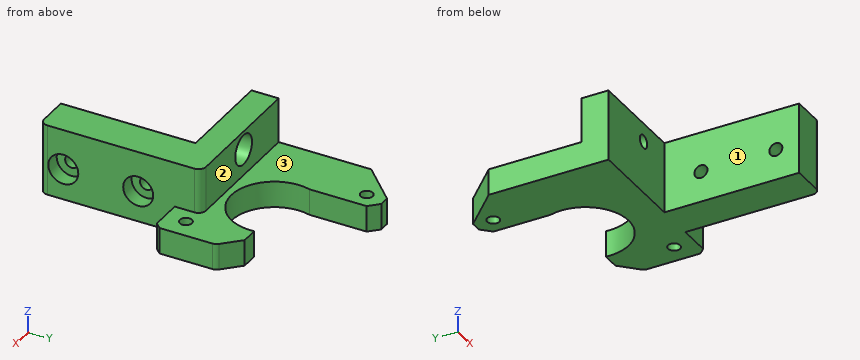
from build123d import *

# Parameters (mm, degrees)
BOSS_EXTRUDE1_DEPTH = 19
BOSS_EXTRUDE2_DEPTH = 7
SKETCH3_R           = 1.75
CUT_EXTRUDE1_DEPTH  = 37.75
SKETCH6_R           = 4
CUT_EXTRUDE4_DEPTH  = 4
SKETCH7_R           = 1.625
CUT_EXTRUDE5_DEPTH  = 20
FILLET1_R           = 2
SKETCH8_R           = 1.75
CUT_EXTRUDE6_DEPTH  = 10
SKETCH9_R           = 4
CUT_EXTRUDE7_DEPTH  = 4


with BuildPart() as part:
    # Sketch1 → Boss-Extrude1 (new body)
    with BuildSketch(Plane.XY):
        Polygon((0, 0), (10, 0), (10, 43.25), (-26.75, 43.25), (-26.75, 36), (0, 36), align=None)
    extrude(amount=BOSS_EXTRUDE1_DEPTH)

    # Sketch2 → Boss-Extrude2 (add)
    with BuildSketch(Plane(origin=(0, 0, 0), x_dir=(-1, 0, 0), z_dir=(0, 0, -1))):
        with BuildLine():
            Line((-10, 36), (26.75, 36))
            Line((26.75, 36), (26.75, 68))
            Line((26.75, 68), (17.25, 77.5))
            Line((17.25, 77.5), (14.5, 77.5))
            Line((14.5, 77.5), (12, 75))
            Line((12, 75), (12, 59.75))
            ThreePointArc((12, 59.75), (2.103531724, 45.089682755), (-10.5, 57.5))
            Line((-10.5, 57.5), (-15, 57.5))
            Line((-15, 57.5), (-20, 52.5))
            Line((-20, 52.5), (-20, 37.5))
            Line((-20, 37.5), (-18.5, 36))
            Line((-18.5, 36), (-10, 36))
        make_face()
    extrude(amount=-BOSS_EXTRUDE2_DEPTH)

    # Sketch3 → Cut-Extrude1 (cut, through all)
    with BuildSketch(Plane(origin=(10, 0, 0), x_dir=(0, 0, -1), z_dir=(1, 0, 0))):
        with Locations((-8.25, 26.25)):
            Circle(SKETCH3_R)
        with Locations((-8.25, 6.25)):
            Circle(SKETCH3_R)
    extrude(amount=-CUT_EXTRUDE1_DEPTH, mode=Mode.SUBTRACT)

    # Sketch6 → Cut-Extrude4 (cut)
    with BuildSketch(Plane(origin=(10, 0, 0), x_dir=(0, 0, -1), z_dir=(1, 0, 0))):
        with Locations((-8.25, 26.25)):
            Circle(SKETCH6_R)
        with Locations((-8.25, 6.25)):
            Circle(SKETCH6_R)
    extrude(amount=-CUT_EXTRUDE4_DEPTH, mode=Mode.SUBTRACT)

    # Sketch7 → Cut-Extrude5 (cut, through all)
    with BuildSketch(Plane(origin=(0, 0, 0), x_dir=(-1, 0, 0), z_dir=(0, 0, -1))):
        with Locations((16.5, 72.5)):
            Circle(SKETCH7_R)
        with Locations((-14.5, 41.5)):
            Circle(SKETCH7_R)
    extrude(amount=-CUT_EXTRUDE5_DEPTH, mode=Mode.SUBTRACT)

    # Fillet1
    fillet1_edges = [part.edges().sort_by_distance(p)[0] for p in [
        (10, 43.25, 13),
        (10, 0, 9.5),
        (20, 52.5, 3.5),
    ]]
    fillet(fillet1_edges, radius=FILLET1_R)

    # Sketch8 → Cut-Extrude6 (cut)
    with BuildSketch(Plane.XZ.offset(-36)):
        with Locations((-10, 14)):
            Circle(SKETCH8_R)
    extrude(amount=-CUT_EXTRUDE6_DEPTH, mode=Mode.SUBTRACT)

    # Sketch9 → Cut-Extrude7 (cut)
    with BuildSketch(Plane(origin=(0, 43.25, 0), x_dir=(1, 0, 0), z_dir=(0, 1, 0))):
        with Locations((-10, -14)):
            Circle(SKETCH9_R)
    extrude(amount=-CUT_EXTRUDE7_DEPTH, mode=Mode.SUBTRACT)


solid = part.part
Verification items for the finished model (mm, model axes). Face numbers are marked on the shaded views. A direction names the side the tool comes from. Give positions to 0.01 mm unless a question says otherwise; leave off trailing zeros. Loops run counter-clockwise (first coordinate to the right, second up) from the corner with the lowest first, then second, coordinate; pieces in that order, holes last.
1) Depth check by flat-ended pin: pin 1 Ø8 at (x, z) = (-10, 8) entering from -Y; pin 2 Ø4 at (x, z) = (-11.5, 3.5) entering from +Y; pin 3 Ø3 at (y, z) = (15.5, 9.5) entering from +X. Enter the tip coordinate at first touch or a pass-through.
2) Sectioned sample at C-C, the plane z = 8.25. Enter the section's corners in (x, y).
3) Sectioned sample at A-A, the plane y = 6.25. Enter the section's corners in (x, z).
4) Thickness scan on line 1 along Y through (x, z) = (7.1, 8.25); line 2 along Y through (x, z) = (-18, 7.75); line 3 along X through (y, z) = (7, 16). Record the ranges inside material, lowest first.
5) Sectioned sample at D-D, the plane x = 9. Enter the section's corners in (y, z), then the cut area to 3 significant figures.
6) Set-up check for the marked faces 1, 2 and 3: record each of +Z, -Z, +X, -X, +Y, -Y from which the full face is reachable in a straight line by a thin tool's end or side.
7) Sectioned sample at B-B, the plane z = 1.75. Enter the section's corners in (x, y) (3 decimals), then the cut area to 3 significant figures.
Answers:
1. pin 1: stops at y = 36
1. pin 2: stops at y = 76.5
1. pin 3: stops at x = 10
2. outline: (-26.75, 36) - (0, 36) - (0, 28) - (6, 28) - (6, 30.25) - (10, 30.25) - (10, 41.25) arc R2 ccw to (8, 43.25) - (-26.75, 43.25) - close; (0, 0) - (8, 0) arc R2 ccw to (10, 2) - (10, 2.25) - (6, 2.25) - (6, 4.5) - (0, 4.5) - close; (0, 8) - (6, 8) - (6, 10.25) - (10, 10.25) - (10, 22.25) - (6, 22.25) - (6, 24.5) - (0, 24.5) - close
3. outline: (0, 0) - (10, 0) - (10, 4.25) - (6, 4.25) - (6, 6.5) - (0, 6.5) - close; (0, 10) - (6, 10) - (6, 12.25) - (10, 12.25) - (10, 19) - (0, 19) - close
4. line 1: y = 0 to 2.25, 10.25 to 22.25, 30.25 to 43.25
4. line 2: y = 36 to 43.25
4. line 3: x = 0 to 10
5. outline: (0.27, 0) - (50.78, 0) - (50.78, 7) - (42.98, 7) - (42.98, 19) - (0.27, 19) - close; hole circle Ø8 at (6.25, 8.25); hole circle Ø8 at (26.25, 8.25)
5. area: 766 mm2
6. face 1: +Z, -Z, -X, -Y
6. face 2: +Z, +X, -X, +Y
6. face 3: +Z, +X, +Y
7. outline: (-26.75, 36) - (0, 36) - (0, 0) - (8, 0) arc R2 ccw to (10, 2) - (10, 36) - (18.5, 36) - (20, 37.5) - (20, 51.672) arc R2 ccw to (19.414, 53.086) - (15, 57.5) - (10.5, 57.5) arc R11.5 cw (long way) to (-12, 59.75) - (-12, 75) - (-14.5, 77.5) - (-17.25, 77.5) - (-26.75, 68) - close; hole circle Ø3.25 at (-16.5, 72.5); hole circle Ø3.25 at (14.5, 41.5)
7. area: 1,350 mm2
